Autodesk Inventor part; units mm, degrees
ref_plane "YZ Plane" through (0, 0, 0) normal (1, 0, 0) x (0, 1, 0)
ref_plane "XZ Plane" through (0, 0, 0) normal (0, 1, 0) x (-1, 0, 0)
ref_plane "XY Plane" through (0, 0, 0) normal (0, 0, 1) x (1, 0, 0)
sketch "スケッチ1" plane through (0, 0, 0) normal (0, 0, 1) x (1, 0, 0)
  line L0 (-75, -215) -> (75, -215)
  line L1 (75, -215) -> (75, 215)
  line L2 (75, 215) -> (-75, 215)
  line L3 (-75, 215) -> (-75, -215)
  line L4 (-75, -215) -> (75, 215) construction
  line L5 (75, -215) -> (-75, 215) construction
  line L6 (-65, -215) -> (-65, 215) construction
  line L7 (-65, 59.8957) -> (59.8957, 65) construction
  line L8 (59.8957, 65) -> (65, -59.8957) construction
  line L9 (65, -59.8957) -> (-59.8957, -65) construction
  line L10 (-59.8957, -65) -> (-65, 59.8957) construction
  line L11 (-65, 59.8957) -> (65, -59.8957) construction
  line L12 (59.8957, 65) -> (-59.8957, -65) construction
  circle A0 centre (-65, 59.8957) radius 2.25
  line L13 (-67.0832, -72.8) -> (72.8, -67.0832) construction
  line L14 (72.8, -67.0832) -> (67.0832, 72.8) construction
  line L15 (67.0832, 72.8) -> (-72.8, 67.0832) construction
  line L16 (-72.8, 67.0832) -> (-67.0832, -72.8) construction
  line L17 (-67.0832, -72.8) -> (67.0832, 72.8) construction
  line L18 (72.8, -67.0832) -> (-72.8, 67.0832) construction
  line L19 (0, 0) -> (0, 70.0584) construction
  circle A1 centre (65, -59.8957) radius 2.25
  circle A2 centre (59.8957, 65) radius 1.6
  circle A3 centre (-59.8957, -65) radius 1.6
  circle A4 centre (0, 0) radius 65
  circle A5 centre (59.8957, 206) radius 1.6
  circle A6 centre (0, 141) radius 65
  circle A7 centre (-65, 200.8957) radius 2.25
  circle A8 centre (-59.8957, 76) radius 1.6
  circle A9 centre (65, 81.1043) radius 2.25
  line L20 (0, 141) -> (0, 211.0584) construction
  circle A10 centre (59.8957, -76) radius 1.6
  circle A11 centre (0, -141) radius 65
  circle A12 centre (-65, -81.1043) radius 2.25
  circle A13 centre (-59.8957, -206) radius 1.6
  circle A14 centre (65, -200.8957) radius 2.25
  line L21 (0, -141) -> (0, -70.9416) construction
  circle A15 centre (59.8957, 65) radius 1.6
  circle A16 centre (0, 0) radius 65
  circle A17 centre (-65, 59.8957) radius 2.25
  circle A18 centre (-59.8957, -65) radius 1.6
  circle A19 centre (65, -59.8957) radius 2.25
  line L22 (0, 0) -> (0, 70.0584) construction
  dimension "d0" = 150
  dimension "d1" = 430
  dimension "d3" = 65
  dimension "d4" = 125
  dimension "d7" = 4.5
  dimension "d8" = 140
  dimension "d9" = 70.0584
  dimension "d10" = 3.2
  dimension "d11" = 130
  dimension "d14" = 141
  dimension "d17" = 141
extrude "押し出し1" add sketch "スケッチ1" along normal blind 3
fillet "フィレット1" radius 3 4 edges at (-75, 215, 1.5) (75, 215, 1.5) (-75, -215, 1.5) (75, -215, 1.5)
properties part number "front_140mm" material "アルミニウム 6061"
Verification items for the finished model (mm, model axes). Coordinates: 2 decimals unless noted, no trailing zeros. Loops run counter-clockwise (first coordinate to the right, second up) from the corner with the lowest first, then second, coordinate; pieces in that order, holes last. Notation, with made-up numbers: (-8.5, 12.25) - (13.5, 12.25) arc R19 cw to (13.5, 44.25) - close; hole circle Ø9 at (69.5, 17). An arc over 180 degrees is marked (long way). Answer as a JSON object with one key per item and string values.
(1) Cross-section at A-A, the plane x = 0. Record the boundary of the cut face in (y, z), then the cut area to 3 significant figures.
Response:
{"outline": "(-215, 0) - (-206, 0) - (-206, 3) - (-215, 3) - close; (-76, 0) - (-65, 0) - (-65, 3) - (-76, 3) - close; (65, 0) - (76, 0) - (76, 3) - (65, 3) - close; (206, 0) - (215, 0) - (215, 3) - (206, 3) - close", "area": "120 mm²"}
(2) Cross-section at B-B, the plane y = 14.5. Record the boundary of the cut face in (x, z).
Response:
{"outline": "(-75, 0) - (-63.36, 0) - (-63.36, 3) - (-75, 3) - close; (63.36, 0) - (75, 0) - (75, 3) - (63.36, 3) - close"}
(3) Cross-section at D-D, the plane x = 43.5. Record the boundary of the cut face in (y, z).
Response:
{"outline": "(-215, 0) - (-189.3, 0) - (-189.3, 3) - (-215, 3) - close; (-92.7, 0) - (-48.3, 0) - (-48.3, 3) - (-92.7, 3) - close; (48.3, 0) - (92.7, 0) - (92.7, 3) - (48.3, 3) - close; (189.3, 0) - (215, 0) - (215, 3) - (189.3, 3) - close"}
(4) Go/stop test with a flat-tipped pin: pin 1 Ø3 at (x, y) = (-59.9, 76) entering from -Z. Record where the tip stops, or that it passes through.
Response:
{"pin 1": "passes through"}
(5) Mould release check, pull along Y, two halves, no side actions. Record for faces 1 (the flat face through (-45, 49, 3)), 2 (the cylindrical face through (34.94, 86.19, 1.48)): pulls with the +Y half, pulls with the -Y half, needs draft (parallel to the pull), parting line crosses it, or undercut.
Response:
{"face 1": "needs draft", "face 2": "undercut"}
(6) Scan lines: line 1 along Y through (x, z) = (-0.5, 2.8); line 2 along Y through (x, z) = (-19, 1.8); line 3 along X through (y, z) = (-127, 0.45). Record each from-to range of solid material in increasing order.
Response:
{"line 1": "y = -215 to -206, -76 to -65, 65 to 76, 206 to 215", "line 2": "y = -215 to -203.16, -78.84 to -62.16, 62.16 to 78.84, 203.16 to 215", "line 3": "x = -75 to -63.47, 63.47 to 75"}
(7) Cross-section at C-C, the plane z = 0.6. Count the separate pieces of the cut face and the enclosed holes in it, then the cut area to 3 significant figures.
Response:
{"separate pieces": "1", "enclosed holes": "15", "area": "24,500 mm²"}
